Check sheet for the drawn part. Datum: minimum x, y, z corner. Units: mm. A direction names the side the tool comes from. Give positions to 0.01 mm unless a question says otherwise; leave off trailing zeros. Loops run counter-clockwise (first coordinate to the right, second up) from the corner with the lowest first, then second, coordinate; pieces in that order, holes last. Notation, with made-up numbers: (-21, -0.5) - (-1, -0.5) arc R13 cw to (-1, 20.5) - close; hole circle Ø4 at (-20, -26). An arc over 180 degrees is marked (long way). Use one line per item in the form item = value.
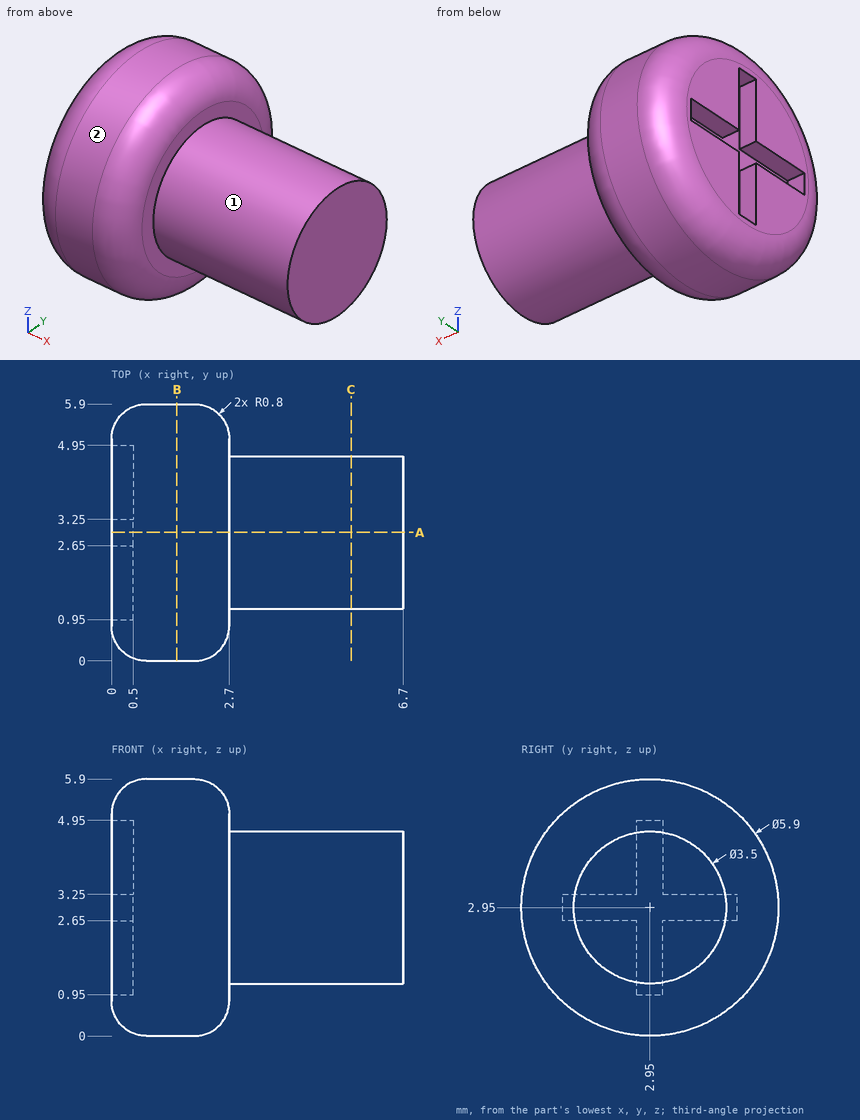
1. Section check B-B, the plane x = 1.5. Record the cut outline in (y, z).
Result set:
outline = circle Ø5.9 at (2.95, 2.95)
2. Section check A-A, the plane y = 2.95. Record the cut outline in (x, z), then the cut area to 3 significant figures.
Result set:
outline = (0, 0.8) arc R0.8 ccw to (0.8, 0) - (1.9, 0) arc R0.8 ccw to (2.7, 0.8) - (2.7, 1.2) - (6.7, 1.2) - (6.7, 4.7) - (2.7, 4.7) - (2.7, 5.1) arc R0.8 ccw to (1.9, 5.9) - (0.8, 5.9) arc R0.8 ccw to (0, 5.1) - (0, 4.95) - (0.5, 4.95) - (0.5, 0.95) - (0, 0.95) - close
area = 27.4 mm²
3. Scan lines: probe 1 along X at (y, z) = (1, 2.15); probe 2 along X at (y, z) = (3, 3.4); probe 3 along Z at (x, y) = (4.25, 1.9). Record each from-to range of solid material in increasing order.
Result set:
probe_1 = 0 to 2.7
probe_2 = 0.5 to 6.7
probe_3 = 1.55 to 4.35
4. Tool access check on the marked faces 1 and 2. Record the directions out of +Z, -Z, +X, -X, +Y, -Y that give a thin tool (end or side, any length) a straight path to the whole face; none if there is none.
Result set:
face_1 = +X
face_2 = +X, -X
5. Section check C-C, the plane x = 5.5. Record the cut outline in (y, z), then the cut area to 3 significant figures.
Result set:
outline = circle Ø3.5 at (2.95, 2.95)
area = 9.62 mm²
6. Depth check by flat-ended pin: pin 1 Ø2 at (x, z) = (4.5, 3.5) entering from -Y; pin 2 Ø2 at (x, y) = (2.5, 4.5) entering from +Z; pin 3 Ø1 at (x, z) = (2.5, 4) entering from +Y. Enter the tip coordinate at first touch or a pass-through.
Result set:
pin_1 = 1.2
pin_2 = 5.81
pin_3 = 5.78
